Part print with two shaded views. Sizes in mm from the minimum x, y, z corner. Round coordinates to 2 decimals unless told otherwise and drop trailing zeros. Loops run counter-clockwise (first coordinate to the right, second up) from the corner with the lowest first, then second, coordinate; pieces in that order, holes last.
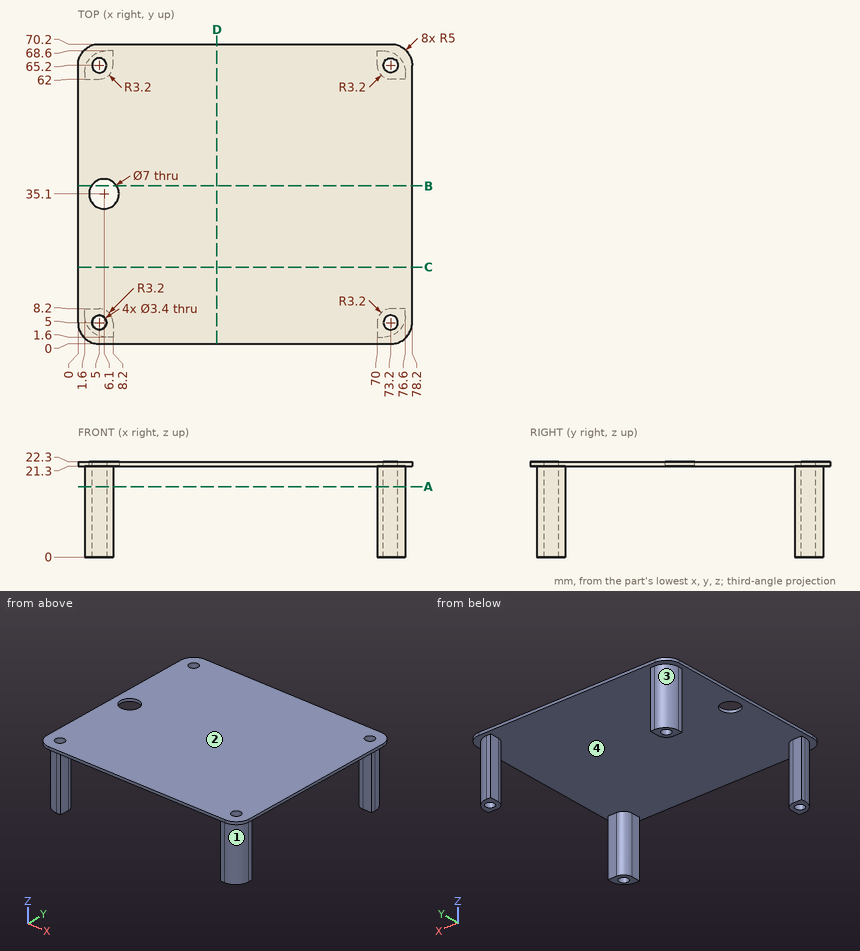
Item 1: Flat gauge pins, fed straight in: P1, Ø3, axis at y = 61, z = 9, coming from the +X side; P2, Ø8, axis at x = 68.5, y = 12, coming from the -Z side; P3, Ø1.7, axis at x = 74.5, z = 10.5, coming from the -Y side. Where does each tip first touch, or does it go through?
Verdict:
P1: stops at x = 76.6
P2: stops at z = 21.3
P3: stops at y = 2.04
Item 2: Mould opens along X. For the marked faces 1, 2, 3 and 4 say: released by +X, released by -X, zero draft, split by the parting line, or undercut.
Verdict:
face 1: released by +X
face 2: zero draft
face 3: released by -X
face 4: undercut
Item 3: Wall check: L1, parallel to Y at x = 73.2, z = 5.75; L2, parallel to Y at x = 4, z = 15.5; L3, parallel to X at y = 5, z = 16.75. Give the ranges that are in metal, low to high.
Verdict:
L1: y = 1.86 to 3.3, 6.7 to 8.2, 62 to 63.5, 66.9 to 68.34
L2: y = 2.33 to 3.63, 6.37 to 8.2, 62 to 63.83, 66.57 to 67.87
L3: x = 1.86 to 3.3, 6.7 to 8.2, 70 to 71.5, 74.9 to 76.34
Item 4: Cut at C-C (y = 18). List the corners of the cut face in (x, z), plus the area to 3 significant figures.
Verdict:
outline: (0, 21.3) - (78.2, 21.3) - (78.2, 22.3) - (0, 22.3) - close
area: 78.2 mm2
Item 5: Cut at A-A (z = 16.5). List the corners of the cut face in (x, y), plus the area to 3 significant figures.
Verdict:
outline: (1.6, 6.6) arc R5 ccw to (6.6, 1.6) - (8.2, 1.6) - (8.2, 5) arc R3.2 ccw to (5, 8.2) - (1.6, 8.2) - close; (1.6, 62) - (5, 62) arc R3.2 ccw to (8.2, 65.2) - (8.2, 68.6) - (6.6, 68.6) arc R5 ccw to (1.6, 63.6) - close; (70, 1.6) - (71.6, 1.6) arc R5 ccw to (76.6, 6.6) - (76.6, 8.2) - (73.2, 8.2) arc R3.2 ccw to (70, 5) - close; (70, 65.2) arc R3.2 ccw to (73.2, 62) - (76.6, 62) - (76.6, 63.6) arc R5 ccw to (71.6, 68.6) - (70, 68.6) - close; hole circle Ø3.4 at (5, 5); hole circle Ø3.4 at (5, 65.2); hole circle Ø3.4 at (73.2, 5); hole circle Ø3.4 at (73.2, 65.2)
area: 108 mm2
Item 6: Cut at D-D (x = 32.5). List the corners of the cut face in (y, z).
Verdict:
outline: (0, 21.3) - (70.2, 21.3) - (70.2, 22.3) - (0, 22.3) - close
Item 7: Cut at B-B (y = 37). List the corners of the cut face in (x, z), plus the area to 3 significant figures.
Verdict:
outline: (0, 21.3) - (3.16, 21.3) - (3.16, 22.3) - (0, 22.3) - close; (9.04, 21.3) - (78.2, 21.3) - (78.2, 22.3) - (9.04, 22.3) - close
area: 72.3 mm2
